from build123d import *

# Parameters (mm, degrees)
SKETCH_W   = 103
SKETCH_H   = 155
SKETCH_R   = 1.275
SKETCH_R_2 = 1.45
SKETCH_R_3 = 1.7
PAD_DEPTH  = 3
FILLET_R   = 20


with BuildPart() as part:
    # Sketch → Pad (new body)
    with BuildSketch(Plane.XY):
        Rectangle(SKETCH_W, SKETCH_H)
        with Locations((-27.5, -72.91422)):
            Circle(SKETCH_R, mode=Mode.SUBTRACT)
        with Locations((27.5, -72.91422)):
            Circle(SKETCH_R, mode=Mode.SUBTRACT)
        with Locations((-20, -2.91422)):
            Circle(SKETCH_R_2, mode=Mode.SUBTRACT)
        with Locations((20, -2.91422)):
            Circle(SKETCH_R_2, mode=Mode.SUBTRACT)
        with Locations((-46.75, 0.08578)):
            Circle(SKETCH_R_3, mode=Mode.SUBTRACT)
        with Locations((-46.75, -72.91422)):
            Circle(SKETCH_R_3, mode=Mode.SUBTRACT)
        with Locations((46.75, -72.91422)):
            Circle(SKETCH_R_3, mode=Mode.SUBTRACT)
        with Locations((46.75, 0.08578)):
            Circle(SKETCH_R_3, mode=Mode.SUBTRACT)
        with Locations((-25, -21.442924)):
            Circle(SKETCH_R_3, mode=Mode.SUBTRACT)
        with Locations((-25, -47.442924)):
            Circle(SKETCH_R_3, mode=Mode.SUBTRACT)
        with Locations((25, -21.442924)):
            Circle(SKETCH_R_3, mode=Mode.SUBTRACT)
        with Locations((25, -47.442924)):
            Circle(SKETCH_R_3, mode=Mode.SUBTRACT)
    extrude(amount=PAD_DEPTH)

    # Fillet
    fillet_edges = [part.edges().sort_by_distance(p)[0] for p in [
        (-51.5, 77.5, 1.5),
        (51.5, 77.5, 1.5),
    ]]
    fillet(fillet_edges, radius=FILLET_R)


solid = part.part
Check sheet for the modelled part. Datum: model origin and axes. Units: mm. Coordinates: 2 decimals unless noted, no trailing zeros. Write each loop counter-clockwise with the first axis right and the second up, starting at its lowest first coordinate (ties: lowest second). Pieces come first, ordered by that corner, then holes.
Item 1: Scan lines: probe 1 along X at (y, z) = (-47.5, 2); probe 2 along Y at (x, z) = (25, 1.35); probe 3 along Y at (x, z) = (27.5, 1.65). Record each from-to range of solid material in increasing order.
Numbers:
probe 1: x = -51.5 to -26.7, -23.3 to 23.3, 26.7 to 51.5
probe 2: y = -77.5 to -49.14, -45.74 to -23.14, -19.74 to 77.5
probe 3: y = -77.5 to -74.19, -71.64 to 77.5
Item 2: Cross-section at A-A on z = 1.75. Count the separate pieces of the cut face and the enclosed holes in it, then the cut area to 3 significant figures.
Numbers:
separate pieces: 1
enclosed holes: 12
area: 15,700 mm2
Item 3: Cross-section at B-B on x = 46.75. Record the boundary of the cut face in (y, z).
Numbers:
outline: (-77.5, 0) - (-74.61, 0) - (-74.61, 3) - (-77.5, 3) - close; (-71.21, 0) - (-1.61, 0) - (-1.61, 3) - (-71.21, 3) - close; (1.79, 0) - (70.44, 0) - (70.44, 3) - (1.79, 3) - close
Item 4: Depth check by flat-ended pin: pin 1 Ø2 at (x, y) = (-25, -47.44) entering from -Z. Enter the tip coordinate at first touch or a pass-through.
Numbers:
pin 1: passes through
Item 5: Mould release check, pull along X, two halves, no side actions. Record for faces 1 (the face through (45.05, 0.16, 1.48)), 2 (the face through (-18.617, -2.479, 1.479)), 3 (the face through (51.5, -11, 1)), 4 (the face through (-45.797, 71.486, 1.521)): released by +X, released by -X, zero draft, split by the parting line, or undercut.
Numbers:
face 1: undercut
face 2: undercut
face 3: released by +X
face 4: released by -X
